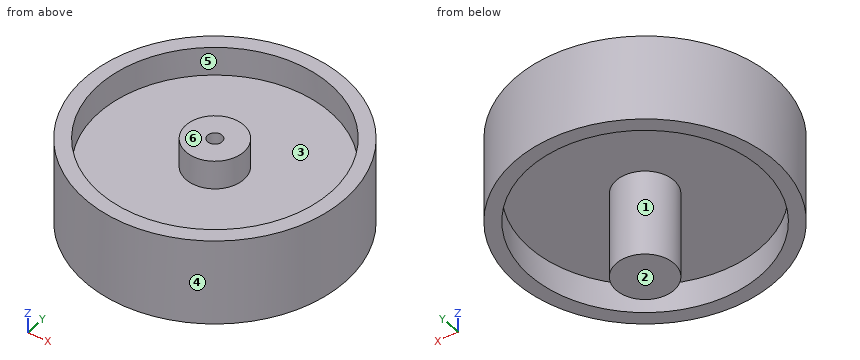
from build123d import *

# Parameters (mm, degrees)
F0_R     = 22.5
F0_R_2   = 20
F1_DEPTH = 15
F0_R_3   = 5
F2_DEPTH = 10
F3_DEPTH = 5
F0_R_4   = 1.25
F4_DEPTH = 25
F5_D     = 2.5
F5_DEPTH = 12
F5_TIP   = 0.7510757738


with BuildPart() as f1:
    # F0 (on Top) → F1 (new body)
    with BuildSketch(Plane.XY):
        Circle(F0_R)
        Circle(F0_R_2, mode=Mode.SUBTRACT)
    extrude(amount=-F1_DEPTH)

    # F0 (on Top) → F2 (join)
    with BuildSketch(Plane.XY):
        Circle(F0_R_2)
        Circle(F0_R_3, mode=Mode.SUBTRACT)
    extrude(amount=-F2_DEPTH)

    # F0 (on Top) → F3 (cut)
    with BuildSketch(Plane.XY):
        Circle(F0_R_2)
        Circle(F0_R_3, mode=Mode.SUBTRACT)
    extrude(amount=-F3_DEPTH, mode=Mode.SUBTRACT)

    # F0 (on Top) → F4 (join)
    with BuildSketch(Plane.XY):
        Circle(F0_R_3)
        Circle(F0_R_4, mode=Mode.SUBTRACT)
        Circle(F0_R_4)
    extrude(amount=-F4_DEPTH)

    # F5
    with Locations(Plane.XY):
        with Locations((0, 0)):
            Hole(F5_D / 2, depth=F5_DEPTH)
            with Locations((0, 0, -(F5_DEPTH + F5_TIP / 2))):  # 118° drill point
                Cone(0, F5_D / 2, F5_TIP, mode=Mode.SUBTRACT)


solid = f1.part
For this review, take the finished solid that the model builds, in its own axes (mm). Face numbers are marked on the shaded views. A direction names the side the tool comes from. Give positions to 0.01 mm unless a question says otherwise; leave off trailing zeros. Write each loop counter-clockwise with the first axis right and the second up, starting at its lowest first coordinate (ties: lowest second). Pieces come first, ordered by that corner, then holes. Notation, with made-up numbers: (-36, -36) -> (-31, -36) arc R14 ccw to (-31, -14) -> close; hole circle Ø5 at (-18.5, -3.75). An arc over 180 degrees is marked (long way). Use CSV: the item, a comma, the result in double quotes.
Q1. Mouldability with a two-part tool opening along Y and no side actions: class the marked faces 4, 5 and 6 as pulls with the +Y half, pulls with the -Y half, needs draft (parallel to the pull), parting line crosses it, or undercut.
Conclusion:
face 4,"parting line crosses it"
face 5,"undercut"
face 6,"needs draft"
Q2. For P1, Ø5, axis at y = 12.5, z = -12, coming from the +X side; P2, Ø1, axis at x = 13, z = -3.5, coming from the +Y side; P3, Ø10, axis at y = 7.5, z = -9.5, coming from the -X side, all flat-tipped, find the tip position at first contact; note any pin that passes through.
Conclusion:
P1,"x = 20.16"
P2,"y = 18.71"
P3,"x = -22.36"
Q3. To check wall thickness, follow probe 1 along Y at (x, z) = (0, -3.35); probe 2 along Y at (x, z) = (1.5, -12.25); probe 3 along X at (y, z) = (-4.5, -3.5). State the ranges of each line that lie inside material, in increasing order. Write a range as [from, to].
Conclusion:
probe 1,"[-22.5, -20], [-5, -1.25], [1.25, 5], [20, 22.5]"
probe 2,"[-22.45, -19.94], [-4.77, 4.77], [19.94, 22.45]"
probe 3,"[-22.05, -19.49], [-2.18, 2.18], [19.49, 22.05]"
Q4. Take a section at C-C, the plane x = -6.5. Write out the cut boundary in (y, z).
Conclusion:
outline,"(-21.54, -15) -> (-18.91, -15) -> (-18.91, -10) -> (18.91, -10) -> (18.91, -15) -> (21.54, -15) -> (21.54, 0) -> (18.91, 0) -> (18.91, -5) -> (-18.91, -5) -> (-18.91, 0) -> (-21.54, 0) -> close"
Q5. Tool access review of the marked faces 1, 2 and 3: name each direction out of +Z, -Z, +X, -X, +Y, -Y from which nothing blocks a thin tool from reaching the whole face with its end or side.
Conclusion:
face 1,"-Z"
face 2,"-Z, +X, -X, +Y, -Y"
face 3,"+Z"
Q6. Take a section at D-D, the plane z = -16.25. Write out the cut boundary in (x, y).
Conclusion:
outline,"circle Ø10 at (0, 0)"
Q7. Take a section at A-A, the plane z = -11.25. Write out the cut boundary in (x, y), then the cut area to 3 significant figures.
Conclusion:
outline,"circle Ø45 at (0, 0); circle Ø10 at (0, 0); hole circle Ø40 at (0, 0); hole circle Ø2.5 at (0, 0)"
area,"407 mm2"
Q8. Take a section at B-B, the plane y = 3. Write out the cut boundary in (x, z).
Conclusion:
outline,"(-22.3, -15) -> (-19.77, -15) -> (-19.77, -10) -> (-4, -10) -> (-4, -25) -> (4, -25) -> (4, -10) -> (19.77, -10) -> (19.77, -15) -> (22.3, -15) -> (22.3, 0) -> (19.77, 0) -> (19.77, -5) -> (4, -5) -> (4, 0) -> (-4, 0) -> (-4, -5) -> (-19.77, -5) -> (-19.77, 0) -> (-22.3, 0) -> close"
